Source: CAD feature listing. Evaluate the final solid. Frame: model axes, mm. A direction names the side the tool comes from. Round coordinates to 2 decimals unless told otherwise and drop trailing zeros. Write each loop counter-clockwise with the first axis right and the second up, starting at its lowest first coordinate (ties: lowest second). Pieces come first, ordered by that corner, then holes. Notation, with made-up numbers: (-26, 3) -> (32, 3) arc R22 ccw to (32, 23) -> close; hole circle Ø6 at (79.5, -18.5). An arc over 180 degrees is marked (long way). Put each result on its own line as item: value.
```python
from build123d import *

# Parameters (mm, degrees)
SKETCH2_R           = 63
BOSS_EXTRUDE2_DEPTH = 4
SKETCH3_R           = 5
CUT_EXTRUDE1_DEPTH  = 4
SKETCH4_R           = 5
SKETCH4_R_2         = 1
BOSS_EXTRUDE3_DEPTH = 14
SKETCH5_R           = 1.5
CUT_EXTRUDE3_DEPTH  = 4
SKETCH7_R           = 1.5
CUT_EXTRUDE6_DEPTH  = 4


with BuildPart() as part:
    # Sketch2 → Boss-Extrude2 (new body)
    with BuildSketch(Plane(origin=(0, 0, 0), x_dir=(1, 0, 0), z_dir=(0, 1, 0))):
        with Locations(Location((0, 0, 0), (0, 0, 270))):
            Circle(SKETCH2_R)
    extrude(amount=BOSS_EXTRUDE2_DEPTH)

    # Sketch3 → Cut-Extrude1 (cut)
    with BuildSketch(Plane(origin=(0, 4, 0), x_dir=(1, 0, 0), z_dir=(0, 1, 0))):
        with Locations(Location((0, 0, 0), (0, 0, 270))):
            Circle(SKETCH3_R)
    extrude(amount=-CUT_EXTRUDE1_DEPTH, mode=Mode.SUBTRACT)

    # Sketch4 → Boss-Extrude3 (add)
    # profile 1 of 3: a face of its own
    with BuildSketch(Plane(origin=(0, 4, 0), x_dir=(1, 0, 0), z_dir=(0, 1, 0))):
        with Locations(Location((-36, 17, 0), (0, 0, 90))):
            Circle(SKETCH4_R)
        with Locations(Location((-36, 17, 0), (0, 0, 90))):
            Circle(SKETCH4_R_2, mode=Mode.SUBTRACT)
    # profile 2 of 3: a face of its own
    with BuildSketch(Plane(origin=(0, 4, 0), x_dir=(1, 0, 0), z_dir=(0, 1, 0))):
        with Locations(Location((36, 17, 0), (0, 0, 90))):
            Circle(SKETCH4_R)
        with Locations(Location((36, 17, 0), (0, 0, 90))):
            Circle(SKETCH4_R_2, mode=Mode.SUBTRACT)
    # profile 3 of 3: a face of its own
    with BuildSketch(Plane(origin=(0, 4, 0), x_dir=(1, 0, 0), z_dir=(0, 1, 0))):
        with Locations(Location((0, -39, 0), (0, 0, 90))):
            Circle(SKETCH4_R)
        with Locations(Location((0, -39, 0), (0, 0, 90))):
            Circle(SKETCH4_R_2, mode=Mode.SUBTRACT)
    extrude(amount=BOSS_EXTRUDE3_DEPTH)

    # Sketch5 → Cut-Extrude3 (cut)
    with BuildSketch(Plane(origin=(0, 4, 0), x_dir=(1, 0, 0), z_dir=(0, 1, 0))):
        with Locations(Location((33.888604279, -21.25, 0), (0, 0, 270))):
            Circle(SKETCH5_R)
        with Locations(Location((-36.099753842, -19.973392205, 0), (0, 0, 270))):
            Circle(SKETCH5_R)
        with Locations(Location((0, 40, 0), (0, 0, 270))):
            Circle(SKETCH5_R)
    extrude(amount=-CUT_EXTRUDE3_DEPTH, mode=Mode.SUBTRACT)

    # Sketch7 → Cut-Extrude6 (cut)
    with BuildSketch(Plane.XZ):
        with Locations(Location((4.063188835, 58.859922668, 0), (0, 0, 270))):
            Circle(SKETCH7_R)
        with Locations(Location((-52.909524673, -26.107129273, 0), (0, 0, 270))):
            Circle(SKETCH7_R)
        with Locations(Location((49.390475327, -32.273533227, 0), (0, 0, 270))):
            Circle(SKETCH7_R)
    extrude(amount=-CUT_EXTRUDE6_DEPTH, mode=Mode.SUBTRACT)


solid = part.part
```
Q1. Cut plane A-A on z = 0. Output: boundary loops of the cut face in (x, y), and give its area (3 significant figures).
Ans:
outline: (-63, 0) -> (-5, 0) -> (-5, 4) -> (-63, 4) -> close; (5, 0) -> (63, 0) -> (63, 4) -> (5, 4) -> close
area: 464 mm^2
Q2. Cut plane D-D on x = 8. Output: boundary loops of the cut face in (y, z), and give its area (3 significant figures).
Ans:
outline: (0, -62.49) -> (4, -62.49) -> (4, 62.49) -> (0, 62.49) -> close
area: 500 mm^2
Q3. Reachability of faces 4 (the cylindrical face through (32.424, 2.028, 20.925)), 5 (the cylindrical face through (0, 11, 44)) from +Z, -Z, +X, -X, +Y, -Y: full face, straight path, thin tool, end or side. Return the list, or none.
Ans:
face 4: +Y, -Y
face 5: +Y
Q4. Cut plane B-B on y = 7. Output: boundary loops of the cut face in (x, z).
Ans:
outline: circle Ø10 at (-36, -17); circle Ø10 at (0, 39); circle Ø10 at (36, -17); hole circle Ø2 at (-36, -17); hole circle Ø2 at (0, 39); hole circle Ø2 at (36, -17)
Q5. Cut plane C-C on z = 36. Output: boundary loops of the cut face in (x, y), and give its area (3 significant figures).
Ans:
outline: (-51.7, 0) -> (51.7, 0) -> (51.7, 4) -> (4, 4) -> (4, 18) -> (-4, 18) -> (-4, 4) -> (-51.7, 4) -> close
area: 526 mm^2
Q6. Material intervals for line 1 (Y direction, x = -52, z = -14); line 2 (Z direction, x = 1, y = 1); line 3 (Z direction, x = 33.5, y = 3), sorted ascending. Write a range as [from, to].
Ans:
line 1: y = [0, 4]
line 2: z = [-62.99, -41.12], [-38.88, -4.9], [4.9, 62.99]
line 3: z = [-53.35, 19.8], [22.7, 53.35]
Q7. Draft query along Z for faces 1 (the cylindrical face through (4.13, 1.97, 60.36)), 2 (the cylindrical face through (-40, 11, -20)), 3 (the flat face through (-1.2, 18, 39.1)). Return one class per face: +Z half, -Z half, draft (parallel to the pull), parting line (faces both ways), or undercut.
Ans:
face 1: undercut
face 2: parting line
face 3: draft
Q8. Pin query (flat end, axial travel): pin 1 (1.5 mm diameter, centred on x = -4.5, y = 10, fed in from +Z); pin 2 (5 mm diameter, centred on x = 33.89, z = 21.25, fed in from +Y); pin 3 (1.5 mm diameter, centred on x = 41, y = 12, fed in from -Z); pin 4 (10 mm diameter, centred on y = 10.5, z = -29.5, fed in from -X). Return the tip coordinate at first contact, or that it passes through.
Ans:
pin 1: stops at z = 42.31
pin 2: stops at y = 4
pin 3: stops at z = -19.63
pin 4: passes through
